```python
from build123d import *

# Parameters (mm, degrees)
CUT_EXTRUDE4_REACH  = 21.219
SKETCH5_R           = 0.79375
SKETCH4_R           = 4
CUT_EXTRUDE3_DEPTH  = 7
BOSS_EXTRUDE1_DEPTH = 10


with BuildPart() as part:
    # Sketch1 → Revolve1 (revolve)
    with BuildSketch(Plane.XY, mode=Mode.PRIVATE) as revolve1_sk:
        Polygon((0, 0), (8.496, 0), (7.5, 15), (3.5, 15), (0, 15), align=None)
    revolve(revolve1_sk.sketch.rotate(Axis((0, 15, 0), (0, -1, 0)), 180), axis=Axis((0, 15, 0), (0, -1, 0)))

    # Sketch5 → Cut-Extrude4 (cut, up to next)
    with BuildSketch(Plane.XZ, mode=Mode.PRIVATE) as cut_extrude4_sk1:
        with Locations((5.401571729, 3.140943396)):
            Circle(SKETCH5_R)
    cut_extrude4_tool1 = extrude(cut_extrude4_sk1.sketch, amount=-CUT_EXTRUDE4_REACH, mode=Mode.PRIVATE) & part.part
    # Sketch5 → Cut-Extrude4 (cut, up to next)
    with BuildSketch(Plane.XZ, mode=Mode.PRIVATE) as cut_extrude4_sk2:
        with Locations((0.019350908, -6.248370036)):
            Circle(SKETCH5_R)
    cut_extrude4_tool2 = extrude(cut_extrude4_sk2.sketch, amount=-CUT_EXTRUDE4_REACH, mode=Mode.PRIVATE) & part.part
    # Sketch5 → Cut-Extrude4 (cut, up to next)
    with BuildSketch(Plane.XZ, mode=Mode.PRIVATE) as cut_extrude4_sk3:
        with Locations((-5.420922637, 3.10742664)):
            Circle(SKETCH5_R)
    cut_extrude4_tool3 = extrude(cut_extrude4_sk3.sketch, amount=-CUT_EXTRUDE4_REACH, mode=Mode.PRIVATE) & part.part
    add(cut_extrude4_tool1.solids().sort_by_distance((5.401572, 0, 3.140943))[0], mode=Mode.SUBTRACT)
    add(cut_extrude4_tool2.solids().sort_by_distance((0.019351, 0, -6.24837))[0], mode=Mode.SUBTRACT)
    add(cut_extrude4_tool3.solids().sort_by_distance((-5.420923, 0, 3.107427))[0], mode=Mode.SUBTRACT)

    # Sketch4 → Cut-Extrude3 (cut)
    with BuildSketch(Plane(origin=(0, 15, 0), x_dir=(1, 0, 0), z_dir=(0, 1, 0))):
        with Locations((0, 7.5)):
            Circle(SKETCH4_R)
        with Locations((6.495190528, -3.75)):
            Circle(SKETCH4_R)
        with Locations((-6.495190528, -3.75)):
            Circle(SKETCH4_R)
    extrude(amount=-CUT_EXTRUDE3_DEPTH, mode=Mode.SUBTRACT)

    # Sketch8 → Boss-Extrude1 (add)
    with BuildSketch(Plane(origin=(0, 15, 0), x_dir=(1, 0, 0), z_dir=(0, 1, 0))):
        with BuildLine():
            Line((1.5, 2.5), (1.5, -2.5))
            ThreePointArc((1.5, -2.5), (3.549509757, 0), (1.5, 2.5))
        make_face()
        with BuildLine():
            Line((-1.5, 2.5), (-1.5, -2.5))
            ThreePointArc((-1.5, -2.5), (-3.549509757, 0), (-1.5, 2.5))
        make_face()
    extrude(amount=BOSS_EXTRUDE1_DEPTH)


solid = part.part
```
Can you work these out from the model? Positions are in its coordinate system, mm. A direction names the side the tool comes from. Give positions to 0.01 mm unless a question says otherwise; leave off trailing zeros. Write each loop counter-clockwise with the first axis right and the second up, starting at its lowest first coordinate (ties: lowest second). Pieces come first, ordered by that corner, then holes. Notation, with made-up numbers: (19, -20.5) - (25, -20.5) arc R12 ccw to (25, -13.5) - close; hole circle Ø8 at (64.25, 67). An arc over 180 degrees is marked (long way). Write item = value, one per line. Start each with the question number.
1. On a 3-axis mill with a long thin cutter (end or side, diameter ignored), from which of +Z, -Z, +X, -X, +Y, -Y can I reach the whole of each face in a straight line? I mean faces 4 (the face through (-2.99, 11.55, 1.82)), 5 (the face through (1.5, 20, 0)), 6 (the face through (0, 8, -5)). Say none if no direction works.
2. Imagine slicing it at C-C (y = 3.5). Please give me the cut outline in (x, z), and give its area (3 significant figures).
3. For pin 1 (1.6 mm diameter, centred on x = 6.5, z = 4, fed in from +Y); pin 2 (10 mm diameter, centred on y = 5.5, z = 1.5, fed in from -X); pin 3 (6 mm diameter, centred on y = 14.5, z = -6, fed in from -X), each with a flat end and sliding along its axis, tell me the tip position at first contact or that it passes through.
4. Imagine slicing it at D-D (y = 6.5). Please give me the cut outline in (x, z).
5. Please list where these lines run through material, in increasing order: line 1 (Y direction, x = 6.25, z = -2.5); line 2 (Y direction, x = 5.25, z = 4); line 3 (X direction, y = 12.75, z = -6).
6. Imagine slicing it at B-B (y = 16.75). Please give me the cut outline in (x, z).
7. Imagine slicing it at A-A (x = 0). Please give me the cut outline in (y, z).
8. Thinking about a two-plate mould opening in Z: for faces 1 (the face through (-0.1, 11.5, -3.5)), 2 (the face through (0, 0, 0)), 3 (the face through (-0.153, 3.944, -7.023)), which applies, released by +Z, released by -Z, zero draft, split by the parting line, or undercut?
Worked answers:
q1.face_4 = +Y
q1.face_5 = +Z, -Z, +Y
q1.face_6 = -Z, +Y
q2.outline = circle Ø16.53 at (0, 0); hole circle Ø1.59 at (-5.42, 3.11); hole circle Ø1.59 at (0.02, -6.25); hole circle Ø1.59 at (5.4, 3.14)
q2.area = 209 mm2
q3.pin_1 = 8
q3.pin_2 = -8.45
q3.pin_3 = -6.93
q4.outline = circle Ø16.13 at (0, 0); hole circle Ø1.59 at (-5.42, 3.11); hole circle Ø1.59 at (0.02, -6.25); hole circle Ø1.59 at (5.4, 3.14)
q5.line_1 = 0 to 15
q5.line_2 = 0 to 8
q5.line_3 = -4.74 to -3.71, 3.71 to 4.74
q6.outline = (-1.5, -2.5) - (-1.5, 2.5) arc R2.55 ccw to start; (1.5, -2.5) arc R2.55 ccw to (1.5, 2.5) - close
q7.outline = (0, -8.5) - (8, -7.96) - (8, -7.04) - (0, -7.04) - close; (0, -5.45) - (8, -5.45) - (8, -3.5) - (15, -3.5) - (15, 7.5) - (0, 8.5) - close
q8.face_1 = released by -Z
q8.face_2 = zero draft
q8.face_3 = undercut
